Verification items for this drawing (mm, ordinates from the low corner). A direction names the side the tool comes from. Round coordinates to 2 decimals unless told otherwise and drop trailing zeros. Order: outer loops, then holes, each group sorted by start corner. A loop starts at its lowest first (then second) coordinate and runs counter-clockwise, first axis right, second up. Notation, with made-up numbers: M 50,18.25 L 103,18.25 A31 cw 103,43.25 Z; hole C 87,-6.5 d10. An arc over 180 degrees is marked long. Return JSON: item names as keys, results as strings. Group by question number.
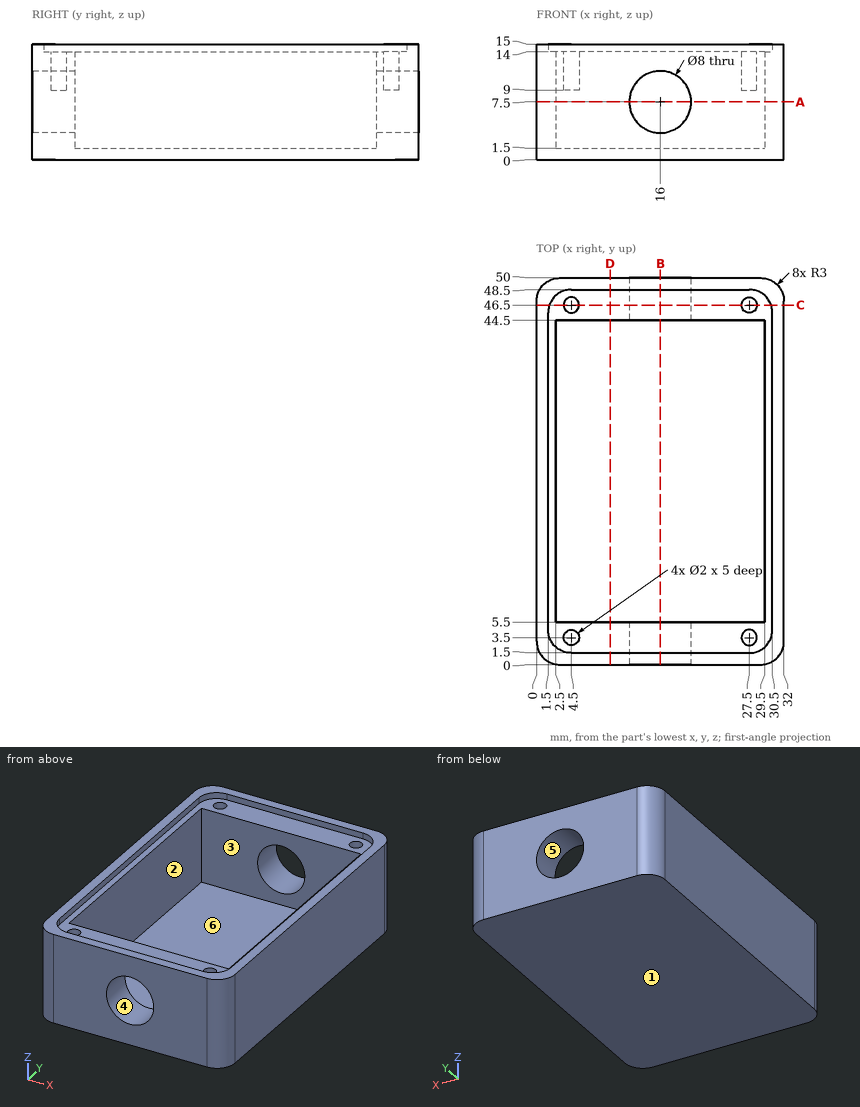
1. Cross-section at B-B (x = 16). Enter the section's corners in (y, z), plus the area to 4 significant figures.
2. Thickness scan on line 1 along X through (y, z) = (46.5, 12.55); line 2 along Y through (x, z) = (4.5, 11.4); line 3 along Y through (x, z) = (26, 11.5). Record the ranges inside material, lowest first. Write a range as from..to.
3. Access from +Z, -Z, +X, -X, +Y, -Y to the whole of each face (thin tool, end or side, straight path). Record for the marked faces 1 and 2.
4. Draft check along Z on the marked faces 3, 4, 5 and 6. Enter one of: +Z half, -Z half, draft (parallel to the pull), parting line (faces both ways), or undercut.
5. Cross-section at C-C (y = 46.5). Enter the section's corners in (x, z).
6. Cross-section at A-A (z = 7.5). Enter the section's corners in (x, y).
7. Go/stop test with flat-tipped pins: pin 1 (8 mm diameter, centred on x = 10.5, y = 10, fed in from +Z); pin 2 (2.5 mm diameter, centred on x = 27.5, y = 3.5, fed in from +Z). Record where each tip stops, or that it passes through.
8. Cross-section at D-D (x = 9.5). Enter the section's corners in (y, z), plus the area to 4 significant figures.
Computed:
{
 "1": {"outline": "M 0,0 L 50,0 L 50,3.5 L 44.5,3.5 L 44.5,1.5 L 5.5,1.5 L 5.5,3.5 L 0,3.5 Z; M 0,11.5 L 5.5,11.5 L 5.5,14 L 1.5,14 L 1.5,15 L 0,15 Z; M 44.5,11.5 L 50,11.5 L 50,15 L 48.5,15 L 48.5,14 L 44.5,14 Z", "area": "127.5 mm²"},
 "2": {"line 1": "x = 0..3.5, 5.5..26.5, 28.5..32", "line 2": "y = 0..2.5, 4.5..5.5, 44.5..45.5, 47.5..50", "line 3": "y = 0..5.5, 44.5..50"},
 "3": {"face 1": "-Z, +X, -X, +Y, -Y", "face 2": "+Z"},
 "4": {"face 3": "draft", "face 4": "undercut", "face 5": "undercut", "face 6": "+Z half"},
 "5": {"outline": "M 0,0 L 32,0 L 32,15 L 30.33,15 L 30.33,14 L 28.5,14 L 28.5,9 L 26.5,9 L 26.5,14 L 5.5,14 L 5.5,9 L 3.5,9 L 3.5,14 L 1.67,14 L 1.67,15 L 0,15 Z; hole C 16,7.5 d8"},
 "6": {"outline": "M 0,3 A3 ccw 3,0 L 12,0 L 12,5.5 L 2.5,5.5 L 2.5,44.5 L 12,44.5 L 12,50 L 3,50 A3 ccw 0,47 Z; M 20,0 L 29,0 A3 ccw 32,3 L 32,47 A3 ccw 29,50 L 20,50 L 20,44.5 L 29.5,44.5 L 29.5,5.5 L 20,5.5 Z"},
 "7": {"pin 1": "stops at z = 1.5", "pin 2": "stops at z = 14"},
 "8": {"outline": "M 0,0 L 50,0 L 50,15 L 48.5,15 L 48.5,14 L 44.5,14 L 44.5,1.5 L 5.5,1.5 L 5.5,14 L 1.5,14 L 1.5,15 L 0,15 Z", "area": "215.5 mm²"}
}
